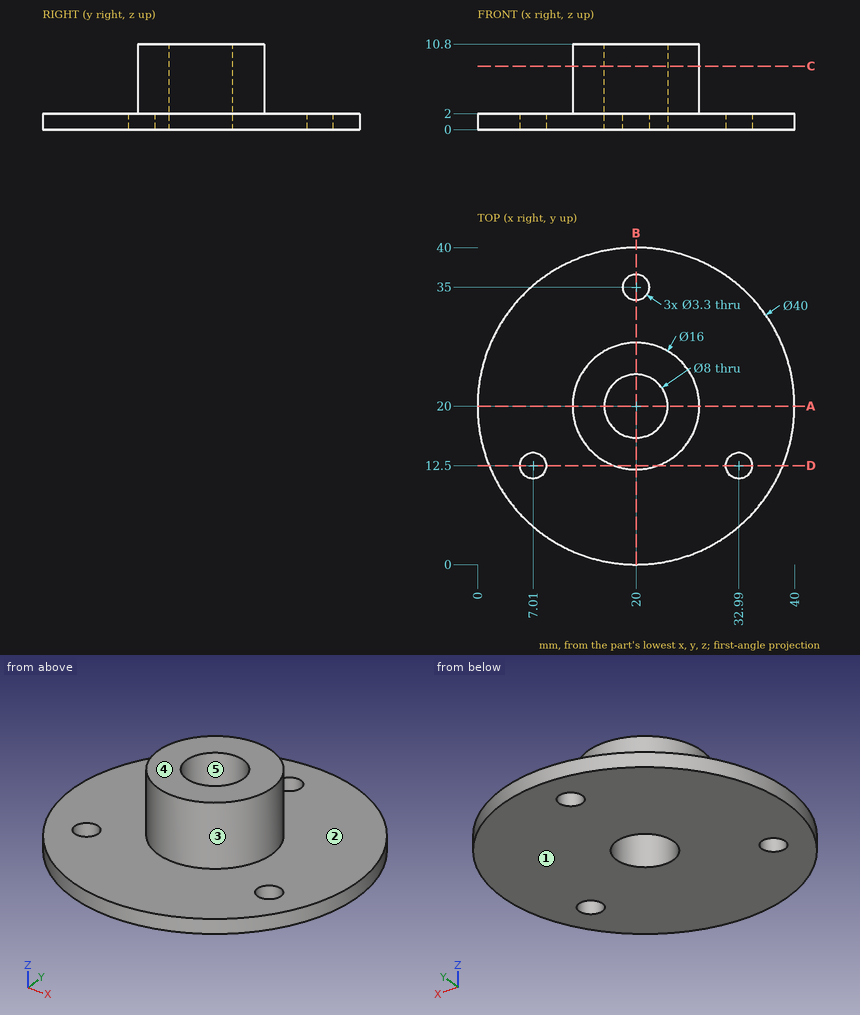
Part print with two shaded views. Sizes in mm from the minimum x, y, z corner. A direction names the side the tool comes from. Give positions to 0.01 mm unless a question says otherwise; leave off trailing zeros. Order: outer loops, then holes, each group sorted by start corner. A loop starts at its lowest first (then second) coordinate and runs counter-clockwise, first axis right, second up. Notation, with made-up numbers: M 12.25,10.25 L 56.25,10.25 A29 cw 56.25,38.25 Z; hole C -6.5,57 d5. An arc over 180 degrees is marked long. Put each result on its own line as item: value.
Item 1: Cut at C-C on z = 8. Write the cut outline in (x, y), then the cut area to 3 significant figures.
Results are:
outline: C 20,20 d16; hole C 20,20 d8
area: 151 mm2
Item 2: Which spindle directions (+Z, -Z, +X, -X, +Y, -Y) get a long thin tool onto all of the face, cutting with end or side? Do the marked faces 1 and 2. Say none if no direction does.
Results are:
face 1: -Z, +X, -X, +Y, -Y
face 2: +Z
Item 3: Wall check: probe 1 along Y at (x, z) = (20, 0.85); probe 2 along Y at (x, z) = (20, 7.5); probe 3 along Z at (x, y) = (24, 4.5). Give the ranges that are in metal, low to high.
Results are:
probe 1: 0 to 16, 24 to 33.35, 36.65 to 40
probe 2: 12 to 16, 24 to 28
probe 3: 0 to 2
Item 4: Cut at A-A on y = 20. Write the cut outline in (x, z).
Results are:
outline: M 0,0 L 16,0 L 16,10.8 L 12,10.8 L 12,2 L 0,2 Z; M 24,0 L 40,0 L 40,2 L 28,2 L 28,10.8 L 24,10.8 Z
Item 5: Drop flat-ended pins along their axis: pin 1 Ø4.5 at (x, y) = (7.01, 12.5) entering from +Z; pin 2 Ø6 at (y, z) = (27.5, 2.5) entering from +X; pin 3 Ø2 at (y, z) = (25, 6) entering from +X. Give the stop position or say it passes through.
Results are:
pin 1: z = 2
pin 2: x = 39.48
pin 3: x = 26.93
Item 6: Pull direction Y, two halves, no side cores. Call the marked faces 3, 4 and 5: +Y half, -Y half, draft (parallel to the pull), parting line (faces both ways), or undercut.
Results are:
face 3: parting line
face 4: draft
face 5: undercut
Item 7: Cut at D-D on y = 12.5. Write the cut outline in (x, z).
Results are:
outline: M 1.46,0 L 5.36,0 L 5.36,2 L 1.46,2 Z; M 8.66,0 L 31.34,0 L 31.34,2 L 22.78,2 L 22.78,10.8 L 17.22,10.8 L 17.22,2 L 8.66,2 Z; M 34.64,0 L 38.54,0 L 38.54,2 L 34.64,2 Z
Item 8: Cut at B-B on x = 20. Write the cut outline in (y, z).
Results are:
outline: M 0,0 L 16,0 L 16,10.8 L 12,10.8 L 12,2 L 0,2 Z; M 24,0 L 33.35,0 L 33.35,2 L 28,2 L 28,10.8 L 24,10.8 Z; M 36.65,0 L 40,0 L 40,2 L 36.65,2 Z
